```python
from build123d import *

# Parameters (mm, degrees)
F0_W          = 48
F0_H          = 24.2
F0_R          = 1.6
F1_DEPTH      = 1
F2_R          = 2.1
F2_W          = 6
F2_H          = 11.3
F3_DEPTH      = 12
F2_W_2        = 4.5
F2_H_2        = 3
F4_DEPTH      = 3.5
F2_R_2        = 1.05
F5_DEPTH      = 2.5
F2_R_3        = 0.75
F6_DEPTH      = 1.001
F7_DEPTH      = 12.001
F7_DEPTH_BACK = 1.001
F2_W_3        = 5.8
F8_DEPTH      = 2.85
F9_R          = 0.5
F10_DEPTH     = 1


with BuildPart() as f1:
    # F0 (on Front) → F1 (new body)
    with BuildSketch(Plane.XZ):
        Rectangle(F0_W, F0_H)
        with Locations((-4.1, -2.4)):
            Circle(F0_R, mode=Mode.SUBTRACT)
        with Locations((9.7, 8.1)):
            Circle(F0_R, mode=Mode.SUBTRACT)
    extrude(amount=-F1_DEPTH)

    # F2 (on face) → F3 (join)
    with BuildSketch(Plane.XZ):
        Polygon((3.4, -6.6), (0.4, -6.6), (0.4, -12.1), (17.8, -12.1), (17.8, -6.6), (7.9, -6.6), (7.9, -9.6), (3.4, -9.6), align=None)
        Polygon((-24, -12.1), (-12.4, -12.1), (-12.4, 0.8), (-12.4, 12.1), (-24, 12.1), align=None)
        with Locations((-21, -8.9)):
            Circle(F2_R, mode=Mode.SUBTRACT)
        with Locations((-21, 2.1)):
            Circle(F2_R, mode=Mode.SUBTRACT)
        Polygon((17.8, -6.6), (17.8, -12.1), (24, -12.1), (24, 12.1), (17.8, 12.1), align=None)
        with Locations((21, -8.9)):
            Circle(F2_R, mode=Mode.SUBTRACT)
        with Locations((21, 2.1)):
            Circle(F2_R, mode=Mode.SUBTRACT)
        with Locations((-3.6, 6.45)):
            Rectangle(F2_W, F2_H)
    extrude(amount=F3_DEPTH)

    # F2 (on face) → F4 (join)
    with BuildSketch(Plane.XZ):
        with Locations((5.65, -8.1)):
            Rectangle(F2_W_2, F2_H_2)
    extrude(amount=F4_DEPTH)

    # F2 (on face) → F5 (join)
    with BuildSketch(Plane.XZ):
        with Locations((7.7, 5.1)):
            Circle(F2_R_2)
    extrude(amount=F5_DEPTH)

    # F2 (on face) → F6 (cut, through all)
    with BuildSketch(Plane.XZ):
        with Locations((15.7, 10.1)):
            Circle(F2_R_3)
    extrude(amount=-F6_DEPTH, mode=Mode.SUBTRACT)

    # F2 (on face) → F7 (cut, two sides)
    with BuildSketch(Plane.XZ) as f7_sk:
        with Locations((-21, 2.1)):
            Circle(F2_R)
        with Locations((21, 2.1)):
            Circle(F2_R)
        with Locations((-21, -8.9)):
            Circle(F2_R)
        with Locations((21, -8.9)):
            Circle(F2_R)
    extrude(amount=F7_DEPTH, mode=Mode.SUBTRACT)
    extrude(f7_sk.sketch, amount=-F7_DEPTH_BACK, mode=Mode.SUBTRACT)

    # F2 (on face) → F8 (join)
    with BuildSketch(Plane.XZ):
        with Locations((-9.5, 6.45)):
            Rectangle(F2_W_3, F2_H)
    extrude(amount=F8_DEPTH)

    # F9 (on face) → F10 (cut)
    with BuildSketch(Plane.XY.offset(12.1)):
        with Locations((-12.4, -7)):
            Circle(F9_R)
    extrude(amount=-F10_DEPTH, mode=Mode.SUBTRACT)


solid = f1.part
```
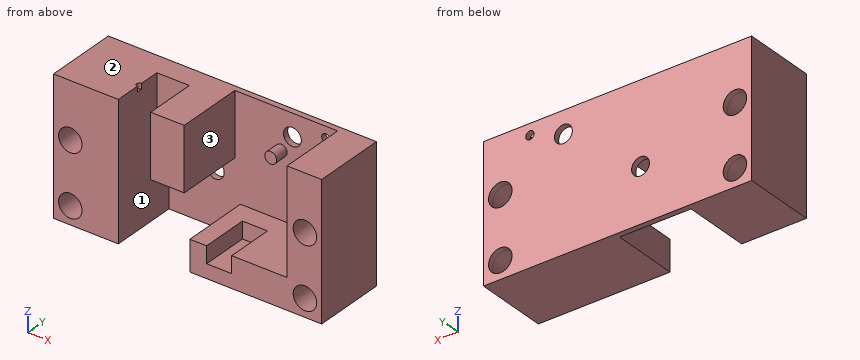
Work out the finished part from the listing and answer in its coordinate system (mm). Face numbers are marked on the shaded views. A direction names the side the tool comes from. Give positions to 0.01 mm unless a question says otherwise; leave off trailing zeros. Order: outer loops, then holes, each group sorted by start corner. A loop starts at its lowest first (then second) coordinate and runs counter-clockwise, first axis right, second up. Notation, with made-up numbers: (27.5, 39.25) - (49.5, 39.25) arc R8 cw to (49.5, 48.25) - close; hole circle Ø6 at (32, -32.5). An arc over 180 degrees is marked (long way). One line per item, written item: value. Start each with the question number.
1. Section B-B, the plane z = -2.4 is taken. Write down the section's boundary in (x, y), then the cut area to 3 significant figures.
2. Section A-A, the plane y = -7 is taken. Write down the section's boundary in (x, z).
3. Which of the six approach directions +Z, -Z, +X, -X, +Y, -Y give full straight-line access (tool end or side, diameter ignored) to the marked faces 1, 2 and 3?
4. Section D-D, the plane z = 1.25 is taken. Write down the section's boundary in (x, y), then the cut area to 3 significant figures.
5. Section C-C, the plane x = 9.7 is taken. Write down the section's boundary in (y, z).
6. Consider line 1 (X direction, y = -9.25, z = 8.5); line 2 (Z direction, x = 21, y = -5.75); line 3 (X direction, y = -7, z = -9). Determine where each line is inside the solid, lowest interval first.
7. Each of these flat-tipped pins is pushed along its axis until it touches: pin 1 Ø12 at (x, z) = (-6.5, -5) entering from -Y; pin 2 Ø5 at (x, y) = (6.5, -6.5) entering from +Z; pin 3 Ø2.5 at (x, z) = (7, 5) entering from -Y. Where does it stop, or does it pass through?
Filled sheet:
1. outline: (-24, -12) - (-12.4, -12) - (-12.4, 0) - (-5.7, 0) - (-5.7, 1) - (-24, 1) - close; (-2.5, 0) - (17.8, 0) - (17.8, -12) - (24, -12) - (24, 1) - (-2.5, 1) - close
1. area: 258 mm²
2. outline: (-24, -12.1) - (-12.4, -12.1) - (-12.4, 11.1) - (-12.9, 11.1) - (-12.9, 12.1) - (-24, 12.1) - close; (-6.6, 0.8) - (-0.6, 0.8) - (-0.6, 12.1) - (-6.6, 12.1) - close; (0.4, -12.1) - (24, -12.1) - (24, 12.1) - (17.8, 12.1) - (17.8, -6.6) - (7.9, -6.6) - (7.9, -9.6) - (3.4, -9.6) - (3.4, -6.6) - (0.4, -6.6) - close; hole circle Ø4.2 at (-21, -8.9); hole circle Ø4.2 at (-21, 2.1); hole circle Ø4.2 at (21, -8.9); hole circle Ø4.2 at (21, 2.1)
3. face 1: -Z, -Y
3. face 2: +Z, +X, -X, +Y, -Y
3. face 3: +Z, -Z, -Y
4. outline: (-24, -12) - (-22.92, -12) - (-22.92, 1) - (-24, 1) - close; (-19.08, -12) - (-12.4, -12) - (-12.4, -2.85) - (-6.6, -2.85) - (-6.6, -12) - (-0.6, -12) - (-0.6, 0) - (17.8, 0) - (17.8, -12) - (19.08, -12) - (19.08, 1) - (-19.08, 1) - close; (22.92, -12) - (24, -12) - (24, 1) - (22.92, 1) - close
4. area: 250 mm²
5. outline: (-12, -12.1) - (1, -12.1) - (1, 6.5) - (0, 6.5) - (0, -6.6) - (-12, -6.6) - close; (0, 9.7) - (1, 9.7) - (1, 12.1) - (0, 12.1) - close
6. line 1: -24 to -12.4, -6.6 to -0.6, 17.8 to 24
6. line 2: -12.1 to -11, -6.8 to 0, 4.2 to 12.1
6. line 3: -24 to -23.1, -18.9 to -12.4, 0.4 to 3.4, 7.9 to 18.9, 23.1 to 24
7. pin 1: y = -12
7. pin 2: z = -6.6
7. pin 3: y = -2.5
